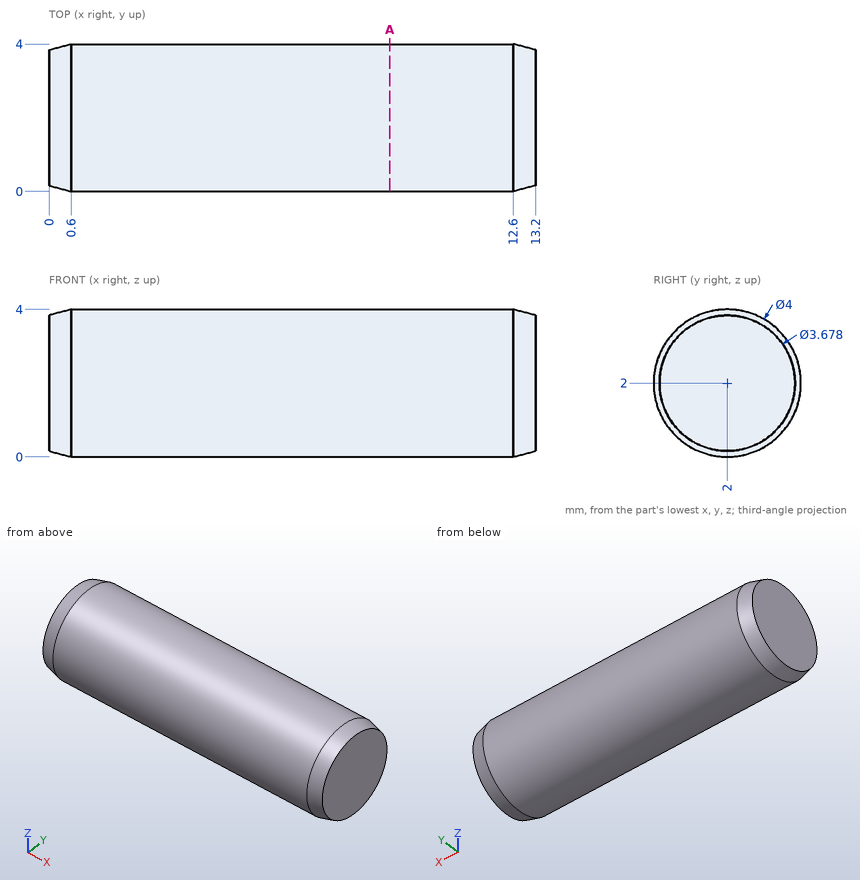
Answer from the drawing. Dimensions are ordinates in mm from the lowest x, y and z of the part. Coordinates: 2 decimals unless noted, no trailing zeros. Write each loop counter-clockwise with the first axis right and the second up, starting at its lowest first coordinate (ties: lowest second). Pieces come first, ordered by that corner, then holes. Notation, with made-up numbers: (16, 38.5) - (62, 38.5) arc R8 cw to (62, 47.5) - close; hole circle Ø3 at (36, 8.25). An arc over 180 degrees is marked (long way). One line per question, with ' | ' between items.
Q1. This flat-tipped pin is pushed along its axis until it touches: P1, Ø1.5, axis at x = 4, z = 1, coming from the +Y side. Where does it stop, or does it pass through?
Result set:
P1: y = 3.98
Q2. Consider L1, parallel to Y at x = 3.5, z = 2.1; L2, parallel to Y at x = 6, z = 3.35 (1 decimal). Determine where each line is inside the solid, lowest interval first. Write a range as [from, to].
Result set:
L1: [0, 4] | L2: [0.5, 3.5]
Q3. Find section A-A, the plane x = 9.25. Write down the section's boundary in (y, z), plus the area to 3 significant figures.
Result set:
outline: circle Ø4 at (2, 2) | area: 12.6 mm^2
